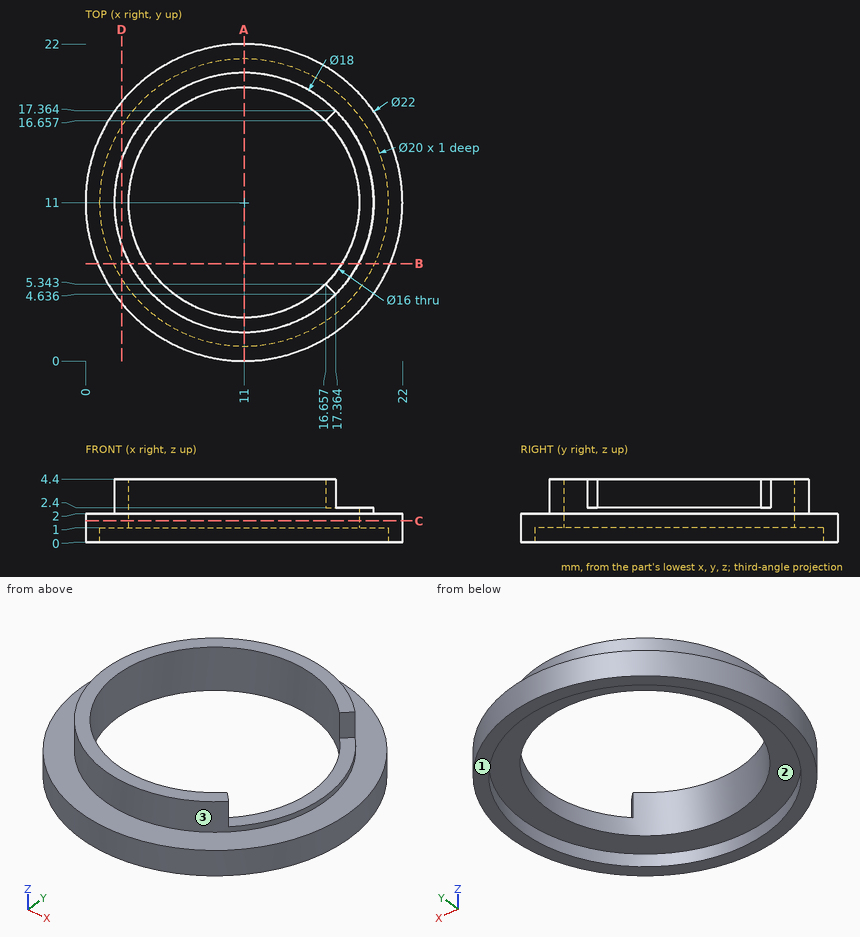
Could you check a few things on this drawing? It's one solid part, dimensions in mm from its lowest x, y, z. A direction names the side the tool comes from. Give positions to 0.01 mm unless a question says otherwise; leave off trailing zeros. Write each loop counter-clockwise with the first axis right and the second up, starting at its lowest first coordinate (ties: lowest second). Pieces come first, ordered by that corner, then holes.
(1) Will these pins go through, and if not, where does the flat tip stop? pin 1 (2 mm diameter, centred on y = 12, z = 2.5, fed in from -X); pin 2 (2.5 mm diameter, centred on x = 18, y = 8.5, fed in from +Z); pin 3 (6 mm diameter, centred on x = 8, y = 11.5, fed in from +Z); pin 4 (1 mm diameter, centred on y = 6.5, z = 2, fed in from +X).
Output values:
pin 1: stops at x = 0
pin 2: stops at z = 2.4
pin 3: passes through
pin 4: stops at x = 21.25
(2) Imagine slicing it at B-B, the plane y = 6.75. Write out the boundary of the cut face in (x, z).
Output values:
outline: (0.85, 0) - (1.95, 0) - (1.95, 1) - (4.22, 1) - (4.22, 4.4) - (3.07, 4.4) - (3.07, 2) - (0.85, 2) - close; (17.78, 1) - (20.05, 1) - (20.05, 0) - (21.15, 0) - (21.15, 2) - (18.93, 2) - (18.93, 2.4) - (17.78, 2.4) - close
(3) Imagine slicing it at C-C, the plane z = 1.5. Write out the boundary of the cut face in (x, y).
Output values:
outline: circle Ø22 at (11, 11); hole circle Ø16 at (11, 11)
(4) Imagine slicing it at A-A, the plane x = 11. Write out the boundary of the cut face in (y, z), and give its area (3 significant figures).
Output values:
outline: (0, 0) - (1, 0) - (1, 1) - (3, 1) - (3, 4.4) - (2, 4.4) - (2, 2) - (0, 2) - close; (19, 1) - (21, 1) - (21, 0) - (22, 0) - (22, 2) - (20, 2) - (20, 4.4) - (19, 4.4) - close
area: 12.8 mm2
(5) If I drill on L1, parallel to Y at x = 11, z = 0.65; L2, parallel to Y at x = 11, z = 2.7; L3, parallel to Z at x = 11.75, y = 19, over which ranges is the centre line in solid material (lowest first)?
Output values:
L1: y = 0 to 1, 21 to 22
L2: y = 2 to 3, 19 to 20
L3: z = 1 to 4.4
(6) On a 3-axis mill with a long thin cutter (end or side, diameter ignored), from which of +Z, -Z, +X, -X, +Y, -Y can I reach the whole of each face in a straight line? I mean the marked faces 1, 2 and 3. Say none if no direction works.
Output values:
face 1: -Z, +X, -X, +Y, -Y
face 2: -Z
face 3: +Z
(7) Imagine slicing it at D-D, the plane x = 2.5. Write out the boundary of the cut face in (y, z).
Output values:
outline: (4.02, 0) - (5.73, 0) - (5.73, 1) - (16.27, 1) - (16.27, 0) - (17.98, 0) - (17.98, 2) - (13.96, 2) - (13.96, 4.4) - (8.04, 4.4) - (8.04, 2) - (4.02, 2) - close
